Autodesk Inventor part; units mm, degrees
ref_plane "YZ Plane" through (0, 0, 0) normal (1, 0, 0) x (0, 1, 0)
ref_plane "XZ Plane" through (0, 0, 0) normal (0, 1, 0) x (-1, 0, 0)
ref_plane "XY Plane" through (0, 0, 0) normal (0, 0, 1) x (1, 0, 0)
sketch "Sketch1" plane through (0, 0, 0) normal (0, 0, 1) x (1, 0, 0)
  circle A0 centre (0, 0) radius 2.8
  dimension "d0" = 5.6
extrude "Extrusion1" add sketch "Sketch1" along normal blind 1.7
fillet "Fillet3" radius 0.5 1 edges at (-2.8, 0, 0)
fillet "Fillet4" radius 1.2 1 edges at (-2.8, 0, 1.7)
sketch "Sketch2" plane through (0, 0, 1.7) normal (0, 0, 1) x (1, 0, 0)
  line L0 (-0.75, -1.299) -> (0.75, -1.299)
  line L1 (0.75, -1.299) -> (1.5, 0)
  line L2 (1.5, 0) -> (0.75, 1.299)
  line L3 (0.75, 1.299) -> (-0.75, 1.299)
  line L4 (-0.75, 1.299) -> (-1.5, 0)
  line L5 (-1.5, 0) -> (-0.75, -1.299)
  dimension "d7" = 3
extrude "Extrusion2" cut sketch "Sketch2" against normal blind 1.7
sketch "Sketch3" plane through (0, 0, 0) normal (0, 1, 0) x (-1, 0, 0)
  line L0 (0, 0) -> (1.5, 0)
  line L1 (2.3, 0) -> (-2.3, 0)
  line L2 (1.5, 0) -> (1.5, 0.8)
  line L3 (1.5, 0.8) -> (0, 0)
  line L4 (0, 0) -> (0, 2.432)
  dimension "d13" = 0
  dimension "d14" = 1.5
  dimension "d15" = 0.8
revolve "Revolution2" add sketch "Sketch3" angle 360 about axis through (0, 0, 0) along (0, 0, 1)
sketch "Sketch4" plane through (0, 0, 0) normal (0, 0, -1) x (-1, 0, 0)
  circle A0 centre (0, 0) radius 2.3
  circle A1 centre (0, 0) radius 1.5
  dimension "d18" = 3
extrude "Extrusion3" add sketch "Sketch4" along normal blind 16 contours A1
thread "Thread1"
properties part number "screw_M3_16_hex"
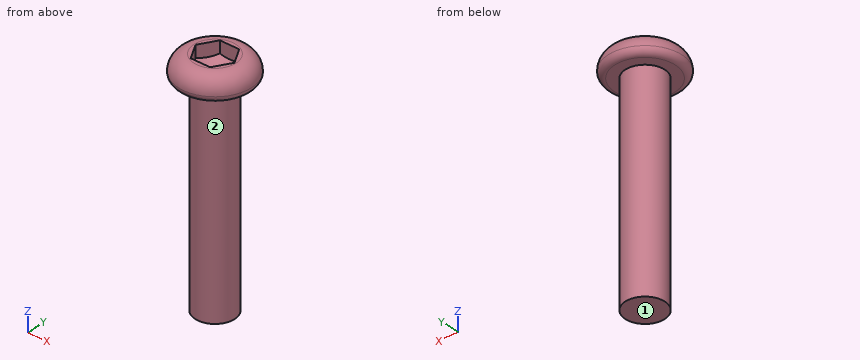
Here's how the part is built. I have some questions about the finished solid (model axes, mm). Face numbers are marked on the shaded views. A direction names the side the tool comes from. Give positions to 0.01 mm unless a question says otherwise; leave off trailing zeros. Loops run counter-clockwise (first coordinate to the right, second up) from the corner with the lowest first, then second, coordinate; pieces in that order, holes last. Notation, with made-up numbers: (65, 8) -> (119, 8) arc R25 cw to (119, 29) -> close; hole circle Ø5 at (-26.5, 69.25). An arc over 180 degrees is marked (long way). Use one line per item in the form item = value. Start each with the question number.
1) Which directions (+Z, -Z, +X, -X, +Y, -Y) give clear straight access to the entire face, cutting with the end or side of a thin tool? Please do the marked faces 1 and 2.
2) Please list where these lines run through material, in increasing order: line 1 along Y through (x, z) = (0.1, -10.5); line 2 along Z through (x, y) = (1.95, -1.1); line 3 along X through (y, z) = (1.15, -6.25).
3) Imagine slicing it at A-A (z = -0.5). Please give me the cut outline in (x, y).
4) For P1, Ø2, axis at y = 1, z = -6, coming from the +X side; P2, Ø3, axis at x = -2, y = 2, coming from the -Z side; P3, Ø1.5, axis at x = -2, y = 2, coming from the -Z side; P4, Ø0.5, axis at x = 0, z = 1, coming from the +Y side, each with a flat end and sliding along its axis, tell me the tip position at first contact or that it passes through.
Check values:
q1.face_1 = -Z, +X, -X, +Y, -Y
q1.face_2 = -Z
q2.line_1 = -1.5 to 1.5
q2.line_2 = 0 to 1.52
q2.line_3 = -0.96 to 0.96
q3.outline = circle Ø3 at (0, 0)
q4.P1 = 1.5
q4.P2 = -16
q4.P3 = 0
q4.P4 = 2.77
